Geometry check sheet. Reference: the model listing, model coordinates, mm. A direction names the side the tool comes from. Coordinates: 2 decimals unless noted, no trailing zeros. Write each loop counter-clockwise with the first axis right and the second up, starting at its lowest first coordinate (ties: lowest second). Pieces come first, ordered by that corner, then holes.
Autodesk Inventor part; units mm, degrees
ref_plane "Work Plane1" through (-30, 0, -90) normal (1, 0, 0) x (0, 0, -1)
ref_plane "Work Plane2" through (-60, 0, -45) normal (0, 0, 1) x (1, 0, 0)
ref_plane "Work Plane3" through (-60, 10, -45) normal (0, 0, 1) x (1, 0, 0)
sketch "Sketch1" plane through (0, 0, 0) normal (0, 1, 0) x (-1, 0, 0)
  line L0 (0, 0) -> (60, 0)
  line L1 (60, 0) -> (60, -90)
  line L2 (60, -90) -> (0, -90)
  line L3 (0, -90) -> (0, 0)
  dimension "d0" = 60
  dimension "d1" = 90
extrude "Extrusion1" add sketch "Sketch1" along normal blind 10
sketch "Sketch2" plane through (0, 10, 0) normal (0, 1, 0) x (1, 0, 0)
  line L0 (0, 20) -> (-60, 20)
  line L1 (0, 70) -> (-60, 70)
  line L2 (-60, 70) -> (-60, 20)
  line L3 (0, 20) -> (0, 70)
  point P0 (0, 0)
extrude "Extrusion2" add sketch "Sketch2" along normal blind 10
sketch "Sketch3" plane through (0, 0, 0) normal (0, -1, 0) x (1, 0, 0)
  line L0 (0, -30) -> (-60, -30)
  line L1 (-60, -30) -> (-60, -60)
  line L2 (0, -90) -> (0, -60)
  line L3 (0, -60) -> (-60, -60)
  line L4 (0, -60) -> (0, -30)
  dimension "d9" = 30
extrude "Extrusion3" cut sketch "Sketch3" against normal blind 10
sketch "Sketch4" plane through (0, 10, 0) normal (0, 1, 0) x (1, 0, 0)
  circle A0 centre (-10, 10) radius 2.75
  circle A1 centre (-50, 10) radius 2.75
  dimension "d13" = 5.5
  dimension "d14" = 5.5
extrude "Extrusion4" cut sketch "Sketch4" against normal blind 10
ref_plane "Work Plane1" through (-30, 0, -90) normal (1, 0, 0) x (0, 0, -1)
sketch "Sketch5" plane through (-30, 0, -90) normal (1, 0, 0) x (0, 0, -1)
  line L0 (-70, 10) -> (-70, 20)
  line L1 (-90, 10) -> (-70, 10)
  line L2 (-70, 20) -> (-90, 10)
  line L3 (-90, 10) -> (-70, 10)
  line L4 (-70, 10) -> (-70, 20)
  point P0 (-90, 0)
extrude "Extrusion5" add sketch "Sketch5" along normal mid plane 4
ref_plane "Work Plane2" through (-60, 0, -45) normal (0, 0, 1) x (1, 0, 0)
mirror "Mirror1" about plane through (-60, 0, -45) normal (0, 0, 1) of "Extrusion4", "Extrusion5"
sketch "Sketch6" plane through (0, 20, 0) normal (0, 1, 0) x (1, 0, 0)
  line L0 (-32, 70) -> (-60, 70)
  line L1 (-40, 20) -> (-40, 70)
  line L2 (-60, 70) -> (-40, 70)
  line L3 (-60, 70) -> (-60, 20)
  line L4 (-60, 20) -> (-40, 20)
  point P0 (0, 0)
  point P1 (0, 20)
extrude "Extrusion6" add sketch "Sketch6" along normal blind 30
fillet "Fillet1" radius 10 2 edges at (-40, 50, -45) (-60, 50, -45)
sketch "Sketch7" plane through (-32, 10, -70) normal (0, 0, -1) x (-1, 0, 0)
  arc A0 (28, 30) -> (8, 30) centre (18, 30) ccw
  circle A1 centre (18, 30) radius 2.75
  point P0 (-32, -10)
  dimension "d24" = 5.5
extrude "Extrusion7" cut sketch "Sketch7" against normal blind 50
ref_plane "Work Plane3" through (-60, 10, -45) normal (0, 0, 1) x (1, 0, 0)
sketch "Sketch8" plane through (-60, 10, -45) normal (0, 0, 1) x (1, 0, 0)
  line L0 (32, 10) -> (60, 10)
  line L1 (60, 10) -> (15.3735, 38.4336)
  arc A0 (20, 30) -> (0, 30) centre (10, 30) ccw
  line L2 (15.3735, 38.4336) -> (15.3735, 10)
  line L3 (15.3735, 10) -> (60, 10)
  point P0 (60, -10)
extrude "Extrusion8" add sketch "Sketch8" along normal mid plane 4
properties part number "MMAE 232 Assignment 1_Part 1 - Dylan Tamras"
1. Gauge pin test, flat ends, axial feed: pin 1 Ø5 at (y, z) = (25, -55.5) entering from +X; pin 2 Ø3 at (y, z) = (14, -77) entering from -X; pin 3 Ø6 at (x, z) = (-44.5, -11.5) entering from +Y. Record the tip position at first contact, or that the pin passes through.
Computed values:
pin 1: stops at x = -40
pin 2: stops at x = -32
pin 3: stops at y = 10
2. Access from +Z, -Z, +X, -X, +Y, -Y to the whole of each face (thin tool, end or side, straight path). Record for faces 1 (the flat face through (-30, 5, -60)), 2 (the cylindrical face through (-45.874, 49.109, -45.35)), 3 (the flat face through (-14, 10, -10)), 4 (the flat face through (-27, 28, -47)), 5 (the flat face through (-49, 25, -20)).
Computed values:
face 1: +X, -X, -Y
face 2: +X, +Y
face 3: +Z, +X, +Y
face 4: -Z, +X, +Y
face 5: +Z, -X, +Y
3. Sectioned sample at A-A, the plane y = 6.5. Record the boundary of the cut face in (x, z), and give its area (3 significant figures).
Computed values:
outline: (-60, -90) - (0, -90) - (0, -60) - (-60, -60) - close; (-60, -30) - (0, -30) - (0, 0) - (-60, 0) - close; hole circle Ø5.5 at (-50, -80); hole circle Ø5.5 at (-50, -10); hole circle Ø5.5 at (-10, -80); hole circle Ø5.5 at (-10, -10)
area: 3,500 mm2
4. Sectioned sample at B-B, the plane z = -10. Record the boundary of the cut face in (x, y), and give its area (3 significant figures).
Computed values:
outline: (-60, 0) - (-52.75, 0) - (-52.75, 10) - (-60, 10) - close; (-47.25, 0) - (-12.75, 0) - (-12.75, 10) - (-28, 10) - (-28, 15) - (-32, 15) - (-32, 10) - (-47.25, 10) - close; (-7.25, 0) - (0, 0) - (0, 10) - (-7.25, 10) - close
area: 510 mm2
5. Draft check along Z on faces 6 (the flat face through (-30, 5, 0)), 7 (the flat face through (-20, 20, -32)), 8 (the flat face through (-30, 10, -45)). Enter one of: released by +Z, released by -Z, zero draft, split by the parting line, or undercut.
Computed values:
face 6: released by +Z
face 7: zero draft
face 8: undercut
6. Sectioned sample at C-C, the plane x = -10. Record the boundary of the cut face in (y, z).
Computed values:
outline: (0, -90) - (10, -90) - (10, -82.75) - (0, -82.75) - close; (0, -77.25) - (10, -77.25) - (10, -70) - (20, -70) - (20, -47) - (26.37, -47) - (26.37, -43) - (20, -43) - (20, -20) - (10, -20) - (10, -12.75) - (0, -12.75) - (0, -30) - (10, -30) - (10, -60) - (0, -60) - close; (0, -7.25) - (10, -7.25) - (10, 0) - (0, 0) - close
7. Thickness scan on line 1 along Z through (x, y) = (-50, 4); line 2 along X through (y, z) = (4.5, -10); line 3 along Y through (x, z) = (-22, -33.5). Record the ranges inside material, lowest first.
Computed values:
line 1: z = -90 to -82.75, -77.25 to -60, -30 to -12.75, -7.25 to 0
line 2: x = -60 to -52.75, -47.25 to -12.75, -7.25 to 0
line 3: y = 10 to 20
